Verification items for the finished model (mm, model axes). Round coordinates to 2 decimals unless told otherwise and drop trailing zeros. Write each loop counter-clockwise with the first axis right and the second up, starting at its lowest first coordinate (ties: lowest second). Pieces come first, ordered by that corner, then holes.
Autodesk Inventor part; units mm, degrees
ref_plane "YZ Plane" through (0, 0, 0) normal (1, 0, 0) x (0, 1, 0)
ref_plane "XZ Plane" through (0, 0, 0) normal (0, 1, 0) x (-1, 0, 0)
sketch "Sketch1" plane through (0, 0, 0) normal (0, 0, 1) x (1, 0, 0)
  circle A0 centre (0, 0) radius 14
  line L0 (0, 0) -> (-50, 0) construction
  circle A1 centre (-50, 0) radius 9
  line L1 (-50.9, 8.9549) -> (-1.4, 13.9298)
  line L2 (-50.9, -8.9549) -> (-1.4, -13.9298)
  point P0 (0, 0)
  dimension "d0" = 18
  dimension "d1" = 28
  dimension "d2" = 50
extrude "Extrusion1" add sketch "Sketch1" along normal mid plane 5
sketch "Sketch2" plane through (0, 0, 2.5) normal (0, 0, 1) x (1, 0, 0)
  arc A0 (-1.4, -13.9298) -> (-1.4, 13.9298) centre (0, 0) ccw
hole "Hole1" at (0, 0, 2.5) direction (0, 0, -1) diameter 15.84 end through all
sketch "Sketch3" plane through (0, 0, 2.5) normal (0, 0, 1) x (1, 0, 0)
  arc A0 (-50.9, 8.9549) -> (-50.9, -8.9549) centre (-50, 0) ccw
hole "Hole2" at (-50, 0, 2.5) direction (0, 0, -1) diameter 9 end through all
properties part number "201-01" material "Steel"
Q1. Depth check by flat-ended pin: P1, Ø9.5, axis at x = 0, y = 0, coming from the +Z side; P2, Ø3, axis at x = -50, y = 3.5, coming from the +Z side; P3, Ø3, axis at x = -33, z = -1.5, coming from the -Y side. Enter the tip coordinate at first touch or a pass-through.
Recorded:
P1: passes through
P2: stops at z = 2.5
P3: stops at y = -10.9
Q2. Sectioned sample at B-B (y = 0). Enter the section's corners in (x, z), plus the area to 3 significant figures.
Recorded:
outline: (-59, -2.5) - (-54.5, -2.5) - (-54.5, 2.5) - (-59, 2.5) - close; (-45.5, -2.5) - (-7.92, -2.5) - (-7.92, 2.5) - (-45.5, 2.5) - close; (7.92, -2.5) - (14, -2.5) - (14, 2.5) - (7.92, 2.5) - close
area: 241 mm2
Q3. Sectioned sample at D-D (z = -0.3). Enter the section's corners in (x, y), plus the area to 3 significant figures.
Recorded:
outline: (-50.9, -8.95) - (-1.4, -13.93) arc R14 ccw (long way) to (-1.4, 13.93) - (-50.9, 8.95) arc R9 ccw to start; hole circle Ø9 at (-50, 0); hole circle Ø15.84 at (0, 0)
area: 1,330 mm2
Q4. Release check for a two-part mould opening along Y. For faces 1 (the flat face through (-26.497, 11.408, -0.035)), 2 (the cylindrical face through (-45.61, 0.98, -0.04)), 3 (the flat face through (-23, 0, -2.5)) record: released by +Y, released by -Y, zero draft, split by the parting line, or undercut.
Recorded:
face 1: released by +Y
face 2: undercut
face 3: zero draft
Q5. Sectioned sample at C-C (y = 5.5). Enter the section's corners in (x, z).
Recorded:
outline: (-57.12, -2.5) - (-5.7, -2.5) - (-5.7, 2.5) - (-57.12, 2.5) - close; (5.7, -2.5) - (12.87, -2.5) - (12.87, 2.5) - (5.7, 2.5) - close
Q6. Sectioned sample at A-A (x = 0). Enter the section's corners in (y, z).
Recorded:
outline: (-14, -2.5) - (-7.92, -2.5) - (-7.92, 2.5) - (-14, 2.5) - close; (7.92, -2.5) - (14, -2.5) - (14, 2.5) - (7.92, 2.5) - close
Q7. Material ranges on line 1 along X through (y, z) = (0, 1.35); line 2 along Y through (x, z) = (0, -1.2); line 3 along X through (y, z) = (-1, -2.1), recorded low to high.
Recorded:
line 1: x = -59 to -54.5, -45.5 to -7.92, 7.92 to 14
line 2: y = -14 to -7.92, 7.92 to 14
line 3: x = -58.94 to -54.39, -45.61 to -7.86, 7.86 to 13.96
